Autodesk Inventor part; units mm, degrees
ref_plane "YZ Plane" through (0, 0, 0) normal (1, 0, 0) x (0, 1, 0)
ref_plane "XZ Plane" through (0, 0, 0) normal (0, 1, 0) x (-1, 0, 0)
ref_plane "XY Plane" through (0, 0, 0) normal (0, 0, 1) x (1, 0, 0)
sketch "Sketch1" plane through (0, 0, 0) normal (0, 1, 0) x (-1, 0, 0)
  arc A0 (-48.5586, 8.5622) -> (49.3077, 0) centre (0, 0) ccw construction
  line L0 (-25, -42.5) -> (25, -42.5) construction
  line L1 (25, -42.5) -> (25, 42.5) construction
  line L2 (25, 42.5) -> (-25, 42.5) construction
  line L3 (-25, -42.5) -> (25, 42.5) construction
  line L4 (25, -42.5) -> (-25, 42.5) construction
  arc A1 (-48.5586, 8.5622) -> (49.3077, 0) centre (0, 0) ccw
  arc A2 (-53.4827, 9.4304) -> (54.3077, 0) centre (0, 0) ccw
  line L5 (-48.5586, 8.5622) -> (-53.4827, 9.4304)
  line L6 (54.3077, 0) -> (49.3077, 0)
  dimension "d0" = 85
  dimension "d1" = 50
  dimension "d2" = 5
  dimension "d4" = 54.3077
  dimension "d5" = 59.535
  dimension "d6" = 170
  dimension "d7" = 42.5
  dimension "d8" = 0
extrude "Extrusion1" add sketch "Sketch1" along normal blind 25 and the other way blind 25
sketch "Sketch2" plane through (0, 0, 0) normal (1, 0, 0) x (0, 1, 0)
  point P0 (0, 0)
sketch "Sketch3" plane through (0, 0, 0) normal (0, 0, 1) x (1, 0, 0)
  line L0 (11.5, -6) -> (-11.5, -6)
  line L1 (-11.5, -6) -> (-11.5, 6)
  line L2 (-11.5, 6) -> (11.5, 6)
  line L3 (11.5, 6) -> (11.5, -6)
  line L4 (11.5, -6) -> (-11.5, 6) construction
  line L5 (-11.5, -6) -> (11.5, 6) construction
  line L6 (15.5, 10) -> (-15.5, 10)
  line L7 (-15.5, 10) -> (-15.5, -10)
  line L8 (-15.5, -10) -> (15.5, -10)
  line L9 (15.5, -10) -> (15.5, 10)
  point P0 (0, 0)
  dimension "d11" = 23
  dimension "d12" = 12
  dimension "d13" = 4
extrude "Extrusion2" add sketch "Sketch3" against normal up to next
sketch "Sketch4" plane through (0, 0, 0) normal (0, 0, 1) x (1, 0, 0)
  line L0 (15.5, 10) -> (-15.5, 10)
  line L1 (-15.5, -10) -> (15.5, -10)
  line L2 (15.5, -10) -> (15.5, 10)
  line L3 (15.5, 10) -> (-15.5, 10)
  line L4 (-15.5, 10) -> (-15.5, -10)
  line L5 (-15.5, -10) -> (15.5, 10) construction
  line L6 (15.5, -10) -> (-15.5, 10) construction
  point P0 (0, 0)
  point P1 (-15.5, 10)
extrude "Extrusion3" cut sketch "Sketch4" against normal blind 25
sketch "Sketch5" plane through (0, 0, 0) normal (0, 1, 0) x (-1, 0, 0)
  point P0 (0, 0)
sketch "Sketch6" plane through (0, 0, 0) normal (0, 0, 1) x (1, 0, 0)
  line L0 (-49.3077, -25) -> (-49.3077, 25)
  line L1 (-49.3077, 7.7599) -> (-49.3077, -14.5309)
  line L2 (53.4827, -25) -> (53.4827, 25)
  line L3 (53.4827, -14.5309) -> (-53.8854, -14.5309)
  line L4 (-49.3077, 2.4805) -> (53.4827, 2.4805)
  line L5 (53.4827, 2.4805) -> (53.4827, -14.5309)
  line L6 (-49.3077, -14.5309) -> (-49.3077, 2.4805)
  line L7 (48.7697, -14.5309) -> (48.5586, 2.4805)
  line L8 (48.5586, -25) -> (48.5586, 25)
  point P0 (0, 0)
  dimension "d24" = 17.0114
  dimension "d25" = 22.5195
  dimension "d26" = 5.2794
  dimension "d27" = 17.0114
chamfer "Chamfer1" distance 1 angle 45 1 edges at (0, -6, -25)
sketch "Sketch7" plane through (0, 0, 0) normal (0, 0, 1) x (1, 0, 0)
  line L0 (-15.5, 10) -> (48.5586, 10)
  line L1 (48.5586, 10) -> (48.5586, 20)
  line L2 (48.5586, -25) -> (48.5586, 25)
  line L3 (48.5586, 20) -> (-49.3077, 20)
  line L4 (-49.3077, 20) -> (-49.3077, 10)
  line L5 (-49.3077, -25) -> (-49.3077, 25)
  line L6 (-15.5, 10) -> (-49.3077, 10)
  point P0 (0, 0)
  dimension "d33" = 10
extrude "Extrusion4" add sketch "Sketch7" against normal up to next
sketch "Sketch8" plane through (15.5, -10, -25) normal (1, 0, 0) x (0, 0, -1)
  line L0 (0, 20) -> (0, 0)
  line L1 (21.8081, 20) -> (21.8081, 0)
  line L2 (0, 11) -> (21.8081, 11)
  line L3 (21.8081, 11) -> (21.8081, 7)
  line L4 (21.8081, 7) -> (0, 7)
  line L5 (0, 7) -> (0, 11)
  point P0 (-25, 10)
  point P1 (0, 16)
  point P2 (0, 3)
  point P3 (0, 7)
  point P4 (21.8081, 11)
  dimension "d36" = 4
  dimension "d39" = 4
extrude "Extrusion5" cut sketch "Sketch8" against normal up to surface (4 mm away)
sketch "Sketch9" plane through (-49.3077, 10, 0) normal (0, -1, 0) x (1, 0, 0)
  circle A0 centre (83.1273, -16.0011) radius 10
  point P0 (49.3077, 0)
  dimension "d42" = 20
  dimension "d43" = 37.4138
extrude "Extrusion6" cut sketch "Sketch9" against normal up to next
sketch "Sketch10" plane through (0, 0, 0) normal (0, 1, 0) x (-1, 0, 0)
  point P0 (0, 0)
ref_plane "Work Plane1" through (-49.3077, 15, 0) normal (0, 1, 0) x (1, 0, 0)
sketch "Sketch11" plane through (-49.3077, 15, 0) normal (0, 1, 0) x (1, 0, 0)
  line L0 (60.1077, 0) -> (60.1077, 16)
  line L1 (60.1077, 16) -> (38.5077, 16)
  line L2 (38.5077, 16) -> (38.5077, 0)
  line L3 (38.5077, -16) -> (60.1077, 16) construction
  line L4 (60.1077, -16) -> (38.5077, 16) construction
  line L5 (97.8663, 0) -> (0, 0)
  line L6 (38.5077, 0) -> (60.1077, 0)
  point P0 (49.3077, 0)
  dimension "d47" = 32
  dimension "d48" = 21.6
  dimension "d49" = 124.019
  dimension "d50" = 55.981
  dimension "d51" = 16
extrude "Extrusion7" cut sketch "Sketch11" along normal up to next
sketch "Sketch12" plane through (-49.3077, 15, 0) normal (0, 1, 0) x (1, 0, 0)
  line L0 (60.1077, 0) -> (38.5077, 0)
  line L1 (38.5077, 0) -> (38.5077, 16)
  line L2 (60.1077, 0) -> (38.5077, 0)
  line L3 (38.5077, 0) -> (38.5077, 4)
  line L4 (38.5077, 4) -> (60.1077, 4)
  line L5 (60.1077, 4) -> (60.1077, 0)
  point P0 (49.3077, 0)
  dimension "d54" = 4
extrude "Extrusion8" cut sketch "Sketch12" against normal up to next
sketch "Sketch13" plane through (-49.3077, 15, 0) normal (0, 1, 0) x (1, 0, 0)
  line L0 (38.5077, 4) -> (60.1077, 4)
  line L1 (60.1077, 16) -> (38.5077, 16)
  line L2 (60.1077, 4) -> (38.5077, 4)
  line L3 (38.5077, 4) -> (38.5077, 16)
  line L4 (38.5077, 16) -> (60.1077, 16)
  line L5 (60.1077, 16) -> (60.1077, 4)
  circle A0 centre (40.8077, 14) radius 1.25
  line L6 (49.3077, 16) -> (49.3077, 4) construction
  circle A1 centre (57.8077, 14) radius 1.25
  point P0 (49.3077, 0)
  dimension "d57" = 2.5
  dimension "d58" = 2.3
  dimension "d59" = 2
extrude "Extrusion9" add sketch "Sketch13" along normal blind 5 contours A0 | A1
properties part number "airframe"
Could you check a few things on this model? Use its own coordinates, in mm. A direction names the side the tool comes from. Give positions to 0.01 mm unless a question says otherwise; leave off trailing zeros. Order: outer loops, then holes, each group sorted by start corner. A loop starts at its lowest first (then second) coordinate and runs counter-clockwise, first axis right, second up. Notation, with made-up numbers: (68, -10.5) - (102, -10.5) arc R17 cw to (102, 14.5) - close; hole circle Ø6 at (-31, 49.5). An arc over 180 degrees is marked (long way). Return JSON: item names as keys, results as strings. Group by question number.
Q1. Thinking about a two-plate mould opening in X: for faces 4 (the face through (0, 25, -51)), 5 (the face through (50.99, -0.35, 8.99)), 6 (the face through (0, 20, -24)), which applies, pulls with the +X half, pulls with the -X half, needs draft (parallel to the pull), parting line crosses it, or undercut?
Q2. Suppose I cut it at D-D, the plane x = -43.5. Please give me the cut outline in (y, z).
Q3. Suppose I cut it at C-C, the plane y = 7.5. Please give me the cut outline in (x, z).
Q4. Suppose I cut it at B-B, the plane y = 18.5. Please give me the cut outline in (x, z), and give its area (3 significant figures).
Q5. Will these pins go through, and if not, where does the flat tip stop? pin 1 Ø10 at (y, z) = (18.5, -43) entering from +X; pin 2 Ø3 at (x, y) = (32.5, 14.5) entering from +Z; pin 3 Ø14.5 at (y, z) = (-0.5, -41.5) entering from -X.
Q6. Which directions (+Z, -Z, +X, -X, +Y, -Y) give clear straight access to the entire face, cutting with the end or side of a thin tool? Please do faces 1 (the face through (8, 20, -14)), 2 (the face through (0, 13, -4)), 3 (the face through (0, -10, -37)).
Q7. Suppose I cut it at A-A, the plane z = -23. Please give me the cut outline in (x, y), and give its area (3 significant figures).
Q8. Please list where these lines run through material, in increasing order: line 1 along X through (y, z) = (7.5, -35); line 2 along Y through (x, z) = (27, -24); line 3 along Y through (x, z) = (1, -29.5). Write a range as [from, to].
Resolved:
{
 "1": {"face 4": "needs draft", "face 5": "pulls with the -X half", "face 6": "undercut"},
 "2": {"outline": "(-25, -32.51) - (25, -32.51) - (25, -23.22) - (20, -23.22) - (20, 0) - (10, 0) - (10, -23.22) - (-25, -23.22) - close"},
 "3": {"outline": "(-54.31, 0) arc R54.31 ccw (long way) to (53.48, 9.43) - (48.56, 8.56) arc R49.31 cw to (15.5, -46.81) - (15.5, -25) - (-15.5, -25) - (-15.5, -46.81) arc R49.31 cw to (-49.31, 0) - close"},
 "4": {"outline": "(-54.31, 0) arc R54.31 ccw (long way) to (53.48, 9.43) - (48.56, 8.56) arc R49.31 cw to (48.56, -8.56) - (48.56, 0) - (10.8, 0) - (10.8, -16) - (-10.8, -16) - (-10.8, 0) - close; circle Ø2.5 at (-8.5, -14); circle Ø2.5 at (8.5, -14); hole circle Ø20 at (33.82, -16)", "area": "4,020 mm2"},
 "5": {"pin 1": "stops at x = 38.8", "pin 2": "stops at z = 0", "pin 3": "stops at x = -42.15"},
 "6": {"face 1": "+Z, +Y", "face 2": "+Z, +Y, -Y", "face 3": "+Z, -Y"},
 "7": {"outline": "(-49.2, -25) - (-43.61, -25) - (-43.61, 10) - (26.68, 10) - (26.68, 20) - (-43.61, 20) - (-43.61, 25) - (-49.2, 25) - close; (40.96, 10) - (43.61, 10) - (43.61, -25) - (49.2, -25) - (49.2, 25) - (43.61, 25) - (43.61, 20) - (40.96, 20) - close", "area": "1,290 mm2"},
 "8": {"line 1": "x = [-41.53, -34.73], [-15.5, 15.5], [34.73, 41.53]", "line 2": "y = [10, 20]", "line 3": "y = [-10, -6], [6, 20]"}
}
